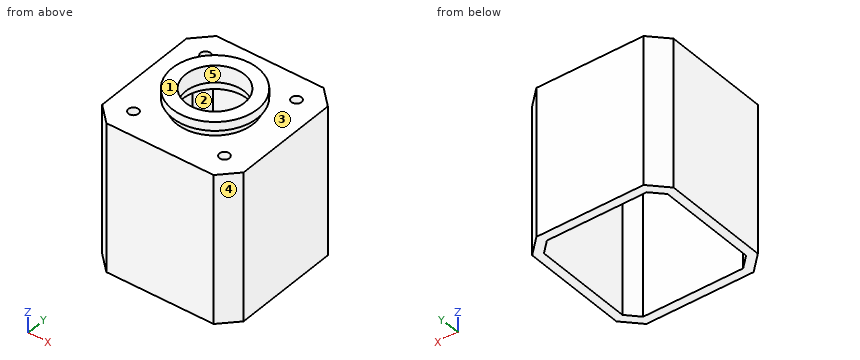
from build123d import *

# Parameters (mm, degrees)
CROQUIS1_R              = 1.7
SALIENTE_EXTRUIR1_DEPTH = 3
CROQUIS17_R             = 11
CORTAR_EXTRUIR7_DEPTH   = 30
CROQUIS19_R             = 13
SALIENTE_EXTRUIR3_DEPTH = 7.25
CROQUIS20_R             = 10
CORTAR_EXTRUIR8_DEPTH   = 14
CORTAR_EXTRUIR9_START   = -1.5
CROQUIS22_R             = 13
CORTAR_EXTRUIR9_DEPTH   = 1.5
SALIENTE_EXTRUIR4_START = -3
CROQUIS23_R             = 14.5
CROQUIS23_R_2           = 13
SALIENTE_EXTRUIR4_DEPTH = 3
SALIENTE_EXTRUIR6_DEPTH = 50.5


with BuildPart() as part:
    # Croquis1 → Saliente-Extruir1 (new body)
    with BuildSketch(Plane.XY):
        Polygon((-20.912159123, -17.544678887), (-21.058605733, 16.394660941), (-17.205052342, 20.455321113), (16.734287486, 20.601767722), (20.794947658, 16.748214331), (20.941394267, -17.191125497), (17.087840877, -21.251785669), (-16.851498951, -21.398232278), align=None)
        with Locations((-15.558605733, 15.101767722)):
            Circle(CROQUIS1_R, mode=Mode.SUBTRACT)
        with Locations((15.441394267, 15.101767722)):
            Circle(CROQUIS1_R, mode=Mode.SUBTRACT)
        with Locations((15.441394267, -15.898232278)):
            Circle(CROQUIS1_R, mode=Mode.SUBTRACT)
        with Locations((-15.558605733, -15.898232278)):
            Circle(CROQUIS1_R, mode=Mode.SUBTRACT)
    extrude(amount=SALIENTE_EXTRUIR1_DEPTH)

    # Croquis17 → Cortar-Extruir7 (cut)
    with BuildSketch(Plane.XY.offset(3)):
        with Locations((-0.058605733, -0.398232278)):
            Circle(CROQUIS17_R)
    extrude(amount=-CORTAR_EXTRUIR7_DEPTH, mode=Mode.SUBTRACT)

    # Croquis19 → Saliente-Extruir3 (add)
    with BuildSketch(Plane.XY.offset(3)):
        with Locations(Location((-0.058605733, -0.398232278, 0), (0, 0, 180))):
            Circle(CROQUIS19_R)
    extrude(amount=SALIENTE_EXTRUIR3_DEPTH)

    # Croquis20 → Cortar-Extruir8 (cut)
    with BuildSketch(Plane.XY.offset(10.25)):
        with Locations((-0.058605733, -0.398232278)):
            Circle(CROQUIS20_R)
    extrude(amount=-CORTAR_EXTRUIR8_DEPTH, mode=Mode.SUBTRACT)

    # Croquis22 → Cortar-Extruir9 (cut)
    with BuildSketch(Plane.XY.offset(10.25).offset(CORTAR_EXTRUIR9_START)):
        with Locations(Location((-0.058605733, -0.398232278, 0), (0, 0, 180))):
            Circle(CROQUIS22_R)
    extrude(amount=CORTAR_EXTRUIR9_DEPTH, mode=Mode.SUBTRACT)

    # Croquis23 → Saliente-Extruir4 (add)
    with BuildSketch(Plane.XY.offset(8.75).offset(SALIENTE_EXTRUIR4_START)):
        with Locations((-0.058605733, -0.398232278)):
            Circle(CROQUIS23_R)
        with Locations(Location((-0.058605733, -0.398232278, 0), (0, 0, 180))):
            Circle(CROQUIS23_R_2, mode=Mode.SUBTRACT)
    extrude(amount=SALIENTE_EXTRUIR4_DEPTH)

    # Croquis25 → Saliente-Extruir6 (add)
    with BuildSketch(Plane.XY.offset(3)):
        Polygon((-24.063774758, 17.586122209), (-18.499196808, 23.44976487), (17.925748755, 23.606936748), (23.789391415, 18.042358797), (23.946563293, -18.382586765), (18.381985343, -24.246229426), (-18.04296022, -24.403401304), (-23.906602881, -18.838823353), align=None)
        Polygon((-20.912159123, -17.544678887), (-16.851498951, -21.398232278), (17.087840877, -21.251785669), (20.941394267, -17.191125497), (20.794947658, 16.748214331), (16.734287486, 20.601767722), (-17.205052342, 20.455321113), (-21.058605733, 16.394660941), align=None, mode=Mode.SUBTRACT)
    extrude(amount=-SALIENTE_EXTRUIR6_DEPTH)


solid = part.part
For this review, take the finished solid that the model builds, in its own axes (mm). Face numbers are marked on the shaded views. A direction names the side the tool comes from. Round coordinates to 2 decimals unless told otherwise and drop trailing zeros. Loops run counter-clockwise (first coordinate to the right, second up) from the corner with the lowest first, then second, coordinate; pieces in that order, holes last. Notation, with made-up numbers: (24, 54.5) - (62, 54.5) arc R19 cw to (62, 58.5) - close; hole circle Ø6 at (-36, -6.75). An arc over 180 degrees is marked (long way). Use one line per item in the form item = value.
Item 1: For line 1 (Y direction, x = 16, z = -43.5); line 2 (Y direction, x = -17, z = -8); line 3 (Z direction, x = 0, y = -13), list the stretches that pass through material, from the lowest coordinate up.
Answers:
line_1 = -24.26 to -21.26, 20.6 to 23.6
line_2 = -24.4 to -21.26, 20.46 to 23.46
line_3 = 0 to 8.75
Item 2: Consider section A-A on z = -41. Write out the cut boundary in (x, y), then the cut area to 3 significant figures.
Answers:
outline = (-24.06, 17.59) - (-23.91, -18.84) - (-18.04, -24.4) - (18.38, -24.25) - (23.95, -18.38) - (23.79, 18.04) - (17.93, 23.61) - (-18.5, 23.45) - close; hole (-21.06, 16.39) - (-20.91, -17.54) - (-16.85, -21.4) - (17.09, -21.25) - (20.94, -17.19) - (20.79, 16.75) - (16.73, 20.6) - (-17.21, 20.46) - close
area = 504 mm^2
Item 3: Consider section D-D on z = 5. Write out the cut boundary in (x, y).
Answers:
outline = circle Ø26 at (-0.06, -0.4); hole circle Ø20 at (-0.06, -0.4)
Item 4: Mouldability with a two-part tool opening along X and no side actions: class the marked faces 3, 4 and 5 as +X half, -X half, draft (parallel to the pull), parting line (faces both ways), or undercut.
Answers:
face_3 = draft
face_4 = +X half
face_5 = undercut
Item 5: Consider section C-C on y = -4. Write out the cut boundary in (x, z).
Answers:
outline = (-23.97, -47.5) - (-20.97, -47.5) - (-20.97, 0) - (-10.45, 0) - (-10.45, 3) - (-9.39, 3) - (-9.39, 8.75) - (-14.1, 8.75) - (-14.1, 5.75) - (-12.55, 5.75) - (-12.55, 3) - (-23.97, 3) - close; (9.27, 3) - (10.34, 3) - (10.34, 0) - (20.88, 0) - (20.88, -47.5) - (23.88, -47.5) - (23.88, 3) - (12.43, 3) - (12.43, 5.75) - (13.99, 5.75) - (13.99, 8.75) - (9.27, 8.75) - close
Item 6: Clearance check with flat-ended pins moving along their axes: P1, Ø12, axis at y = -1.5, z = -10.5, coming from the -X side; P2, Ø1, axis at y = 0, z = -38.5, coming from the +X side; P3, Ø1.5, axis at y = 14, z = 1, coming from the +X side; P4, Ø8, axis at x = 19, y = -4, coming from the -Z side. State where each tip first meets the part, or that it passes through.
Answers:
P1 = -24.01
P2 = 23.87
P3 = 23.81
P4 = -47.5
Item 7: Tool access review of the marked faces 1 and 2: name each direction out of +Z, -Z, +X, -X, +Y, -Y from which nothing blocks a thin tool from reaching the whole face with its end or side.
Answers:
face_1 = +Z, +X, -X, +Y, -Y
face_2 = -Z
Item 8: Consider section B-B on x = 7.5. Write out the cut boundary in (y, z), then the cut area to 3 significant figures.
Answers:
outline = (-24.29, -47.5) - (-21.29, -47.5) - (-21.29, 0) - (-8.39, 0) - (-8.39, 3) - (-6.95, 3) - (-6.95, 8.75) - (-12.77, 8.75) - (-12.77, 5.75) - (-10.97, 5.75) - (-10.97, 3) - (-24.29, 3) - close; (6.15, 3) - (7.59, 3) - (7.59, 0) - (20.56, 0) - (20.56, -47.5) - (23.56, -47.5) - (23.56, 3) - (10.18, 3) - (10.18, 5.75) - (11.98, 5.75) - (11.98, 8.75) - (6.15, 8.75) - close
area = 438 mm^2
